Geometry: final body of the model. Coordinates: model frame, mm. Give positions to 0.01 mm unless a question says otherwise; leave off trailing zeros. Write each loop counter-clockwise with the first axis right and the second up, starting at its lowest first coordinate (ties: lowest second). Pieces come first, ordered by that corner, then holes. Notation, with made-up numbers: (89, -26.75) - (145, -26.75) arc R33 cw to (145, 6.25) - close; hole circle Ø6 at (28.5, 36). An arc over 180 degrees is marked (long way). Return JSON: item names as keys, results as strings.
from build123d import *

# Parameters (mm, degrees)
SKETCH1_R           = 6.35
BOSS_EXTRUDE1_DEPTH = 250
BOSS_EXTRUDE2_DEPTH = 1.5875
CUT_EXTRUDE1_REACH  = 5.175
SKETCH3_R           = 4


with BuildPart() as part:
    # Sketch1 → Boss-Extrude1 (new body, symmetric)
    with BuildSketch(Plane.XY):
        Circle(SKETCH1_R)
    extrude(amount=BOSS_EXTRUDE1_DEPTH, both=True)

    # Sketch2 → Boss-Extrude2 (add, symmetric)
    with BuildSketch(Plane(origin=(0, 0, -250), x_dir=(-1, 0, 0), z_dir=(0, 0, -1))):
        with BuildLine():
            Line((-6.285975, 0.899452), (-14.01986, -53.150124))
            ThreePointArc((-14.01986, -53.150124), (-12.613526, -57.930696), (-8.080356, -60))
            Line((-8.080356, -60), (8.080356, -60))
            ThreePointArc((8.080356, -60), (12.613526, -57.930696), (14.01986, -53.150124))
            Line((14.01986, -53.150124), (6.285975, 0.899452))
            ThreePointArc((6.285975, 0.899452), (0, 6.35), (-6.285975, 0.899452))
        make_face()
    extrude(amount=BOSS_EXTRUDE2_DEPTH, both=True)

    # Sketch3 → Cut-Extrude1 (cut, up to next)
    with BuildSketch(Plane.XY.offset(-248.4125), mode=Mode.PRIVATE) as cut_extrude1_sk1:
        with Locations((-8.080356, -54)):
            Circle(SKETCH3_R)
    cut_extrude1_tool1 = extrude(cut_extrude1_sk1.sketch, amount=-CUT_EXTRUDE1_REACH, mode=Mode.PRIVATE) & part.part
    add(cut_extrude1_tool1.solids().sort_by_distance((-8.080356, -54, -248.4125))[0], mode=Mode.SUBTRACT)
    # Sketch3 → Cut-Extrude1 (cut, up to next)
    with BuildSketch(Plane.XY.offset(-248.4125), mode=Mode.PRIVATE) as cut_extrude1_sk2:
        with Locations((8.080356, -54)):
            Circle(SKETCH3_R)
    cut_extrude1_tool2 = extrude(cut_extrude1_sk2.sketch, amount=-CUT_EXTRUDE1_REACH, mode=Mode.PRIVATE) & part.part
    add(cut_extrude1_tool2.solids().sort_by_distance((8.080356, -54, -248.4125))[0], mode=Mode.SUBTRACT)


solid = part.part
Q1. Section query C-C, the plane y = -29. Return the cut outline in (x, z).
Answer key:
{"outline": "(-10.56, -251.59) - (10.56, -251.59) - (10.56, -248.41) - (-10.56, -248.41) - close"}
Q2. Mould query, pull axis X, two halves, no side actions, for faces 1 (the cylindrical face through (7.2, -57.9, -250)), 2 (the flat face through (10.1, -25.75, -250.02)), 3 (the flat face through (0, 0, 250)), 4 (the cylindrical face through (-8.947, -57.905, -249.978)). Classes: pulls with the +X half, pulls with the -X half, needs draft (parallel to the pull), parting line crosses it, or undercut.
Answer key:
{"face 1": "undercut", "face 2": "pulls with the +X half", "face 3": "needs draft", "face 4": "undercut"}
Q3. Section query B-B, the plane z = -162. Return the cut outline in (x, y).
Answer key:
{"outline": "circle Ø12.7 at (0, 0)"}
Q4. Pin query (flat end, axial travel): P1, Ø4, axis at x = 10.5, y = -39, coming from the +Z side. Return the tip coordinate at first contact, or that it passes through.
Answer key:
{"P1": "stops at z = -248.41"}
Q5. Material intervals for probe 1 along Z at (x, y) = (-10, -42); probe 2 along Y at (x, z) = (-1.25, 191); probe 3 along Y at (x, z) = (3, 225), sorted ascending. Write a range as [from, to].
Answer key:
{"probe 1": "z = [-251.59, -248.41]", "probe 2": "y = [-6.23, 6.23]", "probe 3": "y = [-5.6, 5.6]"}
Q6. Section query A-A, the plane x = 0. Return the cut outline in (y, z).
Answer key:
{"outline": "(-60, -251.59) - (6.35, -251.59) - (6.35, 250) - (-6.35, 250) - (-6.35, -248.41) - (-60, -248.41) - close"}
